from build123d import *

# Parameters (mm, degrees)
SKETCH_1_R        = 2.25
SKETCH_1_R_2      = 1.7
EXTRUDE_259_DEPTH = 8


with BuildPart() as part:
    # 草图1 → Extrude 259 (new body)
    with BuildSketch(Plane.XY):
        Polygon((-24, -20), (-20, -24), (21, -24), (37, -14), (63, -14), (79, -24), (120, -24), (124, -20), (124, 20), (120, 24), (79, 24), (63, 14), (37, 14), (21, 24), (-20, 24), (-24, 20), (-24, 5), (8, 5), (8, -5), (-24, -5), align=None)
        with Locations((-8.85, -8.85)):
            Circle(SKETCH_1_R, mode=Mode.SUBTRACT)
        with Locations((-8.85, 8.85)):
            Circle(SKETCH_1_R, mode=Mode.SUBTRACT)
        with Locations((8.85, -8.85)):
            Circle(SKETCH_1_R, mode=Mode.SUBTRACT)
        with Locations((8.85, 8.85)):
            Circle(SKETCH_1_R, mode=Mode.SUBTRACT)
        with Locations((85.155, -14.845)):
            Circle(SKETCH_1_R_2, mode=Mode.SUBTRACT)
        with Locations((85.155, 14.845)):
            Circle(SKETCH_1_R_2, mode=Mode.SUBTRACT)
        with Locations((114.845, -14.845)):
            Circle(SKETCH_1_R_2, mode=Mode.SUBTRACT)
        with Locations((114.845, 14.845)):
            Circle(SKETCH_1_R_2, mode=Mode.SUBTRACT)
    extrude(amount=EXTRUDE_259_DEPTH)


solid = part.part
Here's how the part is built. I have some questions about the finished solid (model axes, mm). A direction names the side the tool comes from. Coordinates: 2 decimals unless noted, no trailing zeros. Write each loop counter-clockwise with the first axis right and the second up, starting at its lowest first coordinate (ties: lowest second). Pieces come first, ordered by that corner, then holes. Notation, with made-up numbers: (-13.5, 50) - (0.5, 50) arc R11 ccw to (0.5, 68) - close; hole circle Ø2 at (65.5, -13.75). An arc over 180 degrees is marked (long way). Use one line per item in the form item = value.
1) On a 3-axis mill with a long thin cutter (end or side, diameter ignored), from which of +Z, -Z, +X, -X, +Y, -Y can I reach the whole of each face in a straight line? I mean faces 1 (the flat face through (-8, 5, 4)), 2 (the flat face through (29, 19, 4)), 3 (the cylindrical face through (-11.1, -8.8, 3.9)). Say none if no direction works.
Solved:
face_1 = +Z, -Z, -X
face_2 = +Z, -Z, +Y
face_3 = +Z, -Z
2) I need wall thicknesses on line 1 (X direction, y = 9, z = 5) (3 decimals); line 2 (Y direction, x = 3, z = 2.25); line 3 (Y direction, x = 86, z = 5.5). Which ranges of each line are inside material? Lowest first, please.
Solved:
line_1 = -24 to -11.095, -6.605 to 6.605, 11.095 to 124
line_2 = -24 to -5, 5 to 24
line_3 = -24 to -16.32, -13.37 to 13.37, 16.32 to 24
3) Suppose I cut it at A-A, the plane x = -8.85. Write out the boundary of the cut face in (y, z), plus the area to 3 significant figures.
Solved:
outline = (-24, 0) - (-11.1, 0) - (-11.1, 8) - (-24, 8) - close; (-6.6, 0) - (-5, 0) - (-5, 8) - (-6.6, 8) - close; (5, 0) - (6.6, 0) - (6.6, 8) - (5, 8) - close; (11.1, 0) - (24, 0) - (24, 8) - (11.1, 8) - close
area = 232 mm2
4) Suppose I cut it at B-B, the plane y = 8.85. Write out the boundary of the cut face in (x, z), plus the area to 3 significant figures.
Solved:
outline = (-24, 0) - (-11.1, 0) - (-11.1, 8) - (-24, 8) - close; (-6.6, 0) - (6.6, 0) - (6.6, 8) - (-6.6, 8) - close; (11.1, 0) - (124, 0) - (124, 8) - (11.1, 8) - close
area = 1,110 mm2
5) I'm going to push flat-ended pins straight in: P1, Ø4, axis at y = -0.5, z = 3, coming from the -X side; P2, Ø4, axis at x = 51, z = 5.5, coming from the -Y side; P3, Ø2, axis at x = 50, z = 1.5, coming from the +Y side. Where does each tip first touch, or does it pass through?
Solved:
P1 = 8
P2 = -14
P3 = 14
6) Suppose I cut it at D-D, the plane z = 6. Give the number of separate pieces and of enclosed holes in the cut face, plus the area to 3 significant figures.
Solved:
separate_pieces = 1
enclosed_holes = 8
area = 5,810 mm2
7) Thinking about a two-plate mould opening in X: for faces 4 (the flat face through (122, 22, 4)), 5 (the flat face through (49, 0, 0)), 6 (the flat face through (-22, 22, 4)), 7 (the cylindrical face through (84.786, 13.185, 3.944)), which applies, released by +X, released by -X, zero draft, split by the parting line, or undercut?
Solved:
face_4 = released by +X
face_5 = zero draft
face_6 = released by -X
face_7 = undercut
8) Suppose I cut it at C-C, the plane x = 9.5. Write out the boundary of the cut face in (y, z).
Solved:
outline = (-24, 0) - (-11, 0) - (-11, 8) - (-24, 8) - close; (-6.7, 0) - (6.7, 0) - (6.7, 8) - (-6.7, 8) - close; (11, 0) - (24, 0) - (24, 8) - (11, 8) - close
